from build123d import *

# Parameters (mm, degrees)
ESQUISSE1_W                     = 20
ESQUISSE1_H                     = 40
BOSS_EXTRU_1_DEPTH              = 4
ESQUISSE2_W                     = 19
ESQUISSE2_H                     = 39
ENL_V_MAT_EXTRU_1_DEPTH         = 3.5
ESQUISSE3_W                     = 4.5
ESQUISSE3_H                     = 1.5
BOSS_EXTRU_2_DEPTH              = 4.5
ESQUISSE4_W                     = 4.5
ESQUISSE4_H                     = 1.5
BOSS_EXTRU_3_DEPTH              = 4.5
ESQUISSE5_W                     = 4.5
ESQUISSE5_H                     = 1.5
BOSS_EXTRU_4_DEPTH              = 4.5
ESQUISSE6_W                     = 4.5
ESQUISSE6_H                     = 1.5
BOSS_EXTRU_5_DEPTH              = 4.5
ESQUISSE7_W                     = 4.5
ESQUISSE7_H                     = 1.5
ENL_V_MAT_EXTRU_2_DEPTH         = 4.5
ESQUISSE8_W                     = 4.5
ESQUISSE8_H                     = 1.5
ENL_V_MAT_EXTRU_3_DEPTH         = 4.5
ESQUISSE9_W                     = 4.5
ESQUISSE9_H                     = 1.5
ENL_V_MAT_EXTRU_4_DEPTH         = 4.5
ESQUISSE10_W                    = 4.5
ESQUISSE10_H                    = 1.5
ENL_V_MAT_EXTRU_5_DEPTH         = 4.5
ESQUISSE11_W                    = 6
ESQUISSE11_H                    = 2.5
ENL_V_MAT_EXTRU_6_DEPTH         = 0.25
ESQUISSE12_W                    = 1.25
ESQUISSE12_H                    = 2
ESQUISSE13_W                    = 1.25
ESQUISSE13_H                    = 2
ESQUISSE14_W                    = 1.25
ESQUISSE14_H                    = 2
ESQUISSE15_W                    = 1.25
ESQUISSE15_H                    = 2
DIAM_TRE_DU_PER_AGE_1_5_1_5_1_D = 1.5
CHANFREIN1_SIZE                 = 0.707106781
CHANFREIN2_SIZE                 = 1
CONG_1_R                        = 1.5
CONG_2_R                        = 2
CONG_3_R                        = 2.5
CONG_4_R                        = 3


with BuildPart() as part:
    # Esquisse1 → Boss.-Extru.1 (new body)
    with BuildSketch(Plane(origin=(0, 0, 0), x_dir=(1, 0, 0), z_dir=(0, 1, 0))):
        with Locations((22.084435946, -33.026080306)):
            Rectangle(ESQUISSE1_W, ESQUISSE1_H)
    extrude(amount=-BOSS_EXTRU_1_DEPTH)

    # Esquisse2 → Enl_v. mat.-Extru.1 (cut)
    with BuildSketch(Plane(origin=(0, 0, 0), x_dir=(-1, 0, 0), z_dir=(0, 1, 0))):
        with Locations((-22.084435946, 33.026080306)):
            Rectangle(ESQUISSE2_W, ESQUISSE2_H)
    extrude(amount=-ENL_V_MAT_EXTRU_1_DEPTH, mode=Mode.SUBTRACT)

    # Esquisse3 → Boss.-Extru.2 (add)
    with BuildSketch(Plane(origin=(12.584435946, 0, 0), x_dir=(0, 0, -1), z_dir=(1, 0, 0))):
        with Locations((-15.776080306, -2.75)):
            Rectangle(ESQUISSE3_W, ESQUISSE3_H)
    extrude(amount=BOSS_EXTRU_2_DEPTH)

    # Esquisse4 → Boss.-Extru.3 (add)
    with BuildSketch(Plane.XY.offset(13.526080306)):
        with Locations((29.334435946, -2.75)):
            Rectangle(ESQUISSE4_W, ESQUISSE4_H)
    extrude(amount=BOSS_EXTRU_3_DEPTH)

    # Esquisse5 → Boss.-Extru.4 (add)
    with BuildSketch(Plane(origin=(12.584435946, 0, 0), x_dir=(0, 0, -1), z_dir=(1, 0, 0))):
        with Locations((-50.276080306, -2.75)):
            Rectangle(ESQUISSE5_W, ESQUISSE5_H)
    extrude(amount=BOSS_EXTRU_4_DEPTH)

    # Esquisse6 → Boss.-Extru.5 (add)
    with BuildSketch(Plane(origin=(0, 0, 52.526080306), x_dir=(-1, 0, 0), z_dir=(0, 0, -1))):
        with Locations((-29.334435946, -2.75)):
            Rectangle(ESQUISSE6_W, ESQUISSE6_H)
    extrude(amount=BOSS_EXTRU_5_DEPTH)

    # Esquisse7 → Enl_v. mat.-Extru.2 (cut)
    with BuildSketch(Plane.ZY.offset(-12.084435946)):
        with Locations((15.276080306, -3.25)):
            Rectangle(ESQUISSE7_W, ESQUISSE7_H)
    extrude(amount=-ENL_V_MAT_EXTRU_2_DEPTH, mode=Mode.SUBTRACT)

    # Esquisse8 → Enl_v. mat.-Extru.3 (cut)
    with BuildSketch(Plane(origin=(0, 0, 13.026080306), x_dir=(-1, 0, 0), z_dir=(0, 0, -1))):
        with Locations((-29.834435946, -3.25)):
            Rectangle(ESQUISSE8_W, ESQUISSE8_H)
    extrude(amount=-ENL_V_MAT_EXTRU_3_DEPTH, mode=Mode.SUBTRACT)

    # Esquisse9 → Enl_v. mat.-Extru.4 (cut)
    with BuildSketch(Plane.ZY.offset(-12.084435946)):
        with Locations((50.776080306, -3.25)):
            Rectangle(ESQUISSE9_W, ESQUISSE9_H)
    extrude(amount=-ENL_V_MAT_EXTRU_4_DEPTH, mode=Mode.SUBTRACT)

    # Esquisse10 → Enl_v. mat.-Extru.5 (cut)
    with BuildSketch(Plane(origin=(32.084435946, 0, 0), x_dir=(0, 0, -1), z_dir=(1, 0, 0))):
        with Locations((-50.776080306, -3.25)):
            Rectangle(ESQUISSE10_W, ESQUISSE10_H)
    extrude(amount=-ENL_V_MAT_EXTRU_5_DEPTH, mode=Mode.SUBTRACT)

    # Esquisse11 → Enl_v. mat.-Extru.6 (cut)
    with BuildSketch(Plane.XY.offset(53.026080306)):
        with Locations((22.084435946, -1.25)):
            Rectangle(ESQUISSE11_W, ESQUISSE11_H)
    extrude(amount=-ENL_V_MAT_EXTRU_6_DEPTH, mode=Mode.SUBTRACT)

    # Esquisse12 → R_volution1 (revolve)
    with BuildSketch(Plane.XY.offset(15.026080306), mode=Mode.PRIVATE) as r_volution1_sk:
        with Locations((30.709435946, -1)):
            Rectangle(ESQUISSE12_W, ESQUISSE12_H)
    revolve(r_volution1_sk.sketch.rotate(Axis((30.084435946, 0, 15.026080306), (0, -1, 0)), 270), axis=Axis((30.084435946, 0, 15.026080306), (0, -1, 0)))

    # Esquisse13 → R_volution2 (revolve)
    with BuildSketch(Plane.XY.offset(15.026080306), mode=Mode.PRIVATE) as r_volution2_sk:
        with Locations((14.709435946, -1)):
            Rectangle(ESQUISSE13_W, ESQUISSE13_H)
    revolve(r_volution2_sk.sketch.rotate(Axis((14.084435946, 0, 15.026080306), (0, -1, 0)), 270), axis=Axis((14.084435946, 0, 15.026080306), (0, -1, 0)))

    # Esquisse14 → R_volution3 (revolve)
    with BuildSketch(Plane.XY.offset(51.026080306), mode=Mode.PRIVATE) as r_volution3_sk:
        with Locations((14.709435946, -1)):
            Rectangle(ESQUISSE14_W, ESQUISSE14_H)
    revolve(r_volution3_sk.sketch.rotate(Axis((14.084435946, 0, 51.026080306), (0, -1, 0)), 270), axis=Axis((14.084435946, 0, 51.026080306), (0, -1, 0)))

    # Esquisse15 → R_volution4 (revolve)
    with BuildSketch(Plane.XY.offset(51.026080306), mode=Mode.PRIVATE) as r_volution4_sk:
        with Locations((30.709435946, -1)):
            Rectangle(ESQUISSE15_W, ESQUISSE15_H)
    revolve(r_volution4_sk.sketch.rotate(Axis((30.084435946, 0, 51.026080306), (0, -1, 0)), 270), axis=Axis((30.084435946, 0, 51.026080306), (0, -1, 0)))

    # Diam_tre du per_age _1.5 _1.5_1 (through all)
    with Locations(Plane(origin=(0, -2.5, 0), x_dir=(-1, 0, 0), z_dir=(0, -1, 0))):
        with Locations((-30.084435946, -51.026080306), (-14.084435946, -51.026080306), (-14.084435946, -15.026080306), (-30.084435946, -15.026080306)):
            Hole(DIAM_TRE_DU_PER_AGE_1_5_1_5_1_D / 2)

    # Chanfrein1
    chanfrein1_edges = [part.edges().sort_by_distance(p)[0] for p in [
        (12.584435946, -3.5, 33.026080306),
        (22.084435946, -3.5, 13.526080306),
        (22.084435946, -3.5, 52.526080306),
        (31.584435946, -3.5, 33.026080306),
    ]]
    chamfer(chanfrein1_edges, length=CHANFREIN1_SIZE)

    # Chanfrein2
    chanfrein2_edges = [part.edges().sort_by_distance(p)[0] for p in [
        (22.084435946, -4, 53.026080306),
        (32.084435946, -4, 33.026080306),
        (12.084435946, -4, 33.026080306),
        (22.084435946, -4, 13.026080306),
    ]]
    chamfer(chanfrein2_edges, length=CHANFREIN2_SIZE)

    # Cong_1
    cong_1_edges = [part.edges().sort_by_distance(p)[0] for p in [
        (12.584435946, -1, 13.526080306),
        (31.584435946, -1, 13.526080306),
        (12.584435946, -1, 52.526080306),
        (31.584435946, -1, 52.526080306),
    ]]
    fillet(cong_1_edges, radius=CONG_1_R)

    # Cong_2
    cong_2_edges = [part.edges().sort_by_distance(p)[0] for p in [
        (12.084435946, -1.25, 53.026080306),
        (32.084435946, -1.25, 53.026080306),
        (12.084435946, -1.25, 13.026080306),
        (32.084435946, -1.25, 13.026080306),
    ]]
    fillet(cong_2_edges, radius=CONG_2_R)

    # Cong_3
    cong_3_edges = [part.edges().sort_by_distance(p)[0] for p in [
        (27.584435946, -3.25, 17.526080306),
        (16.584435946, -3.25, 48.526080306),
        (27.584435946, -3.25, 48.526080306),
        (16.584435946, -3.25, 17.526080306),
    ]]
    fillet(cong_3_edges, radius=CONG_3_R)

    # Cong_4
    cong_4_edges = [part.edges().sort_by_distance(p)[0] for p in [
        (17.084435946, -2.75, 18.026080306),
        (27.084435946, -2.75, 18.026080306),
        (17.084435946, -2.75, 48.026080306),
        (27.084435946, -2.75, 48.026080306),
    ]]
    fillet(cong_4_edges, radius=CONG_4_R)


solid = part.part
Verification items for the finished model (mm, model axes). A direction names the side the tool comes from. Give positions to 0.01 mm unless a question says otherwise; leave off trailing zeros. Loops run counter-clockwise (first coordinate to the right, second up) from the corner with the lowest first, then second, coordinate; pieces in that order, holes last. Notation, with made-up numbers: (78.5, 55.25) - (83.5, 55.25) arc R19 cw to (83.5, 87.25) - close; hole circle Ø7 at (-16, 5). An arc over 180 degrees is marked (long way). Write item = value, one per line. Start each with the question number.
Q1. Cross-section at B-B, the plane z = 30. Enter the section's corners in (x, y), and give its area (3 significant figures).
Q2. Mould release check, pull along Z, two halves, no side actions. Record for faces 1 (the face through (22, -1, 13.026)), 2 (the face through (22.007, -3.507, 52.519)), 3 (the face through (17.084, -3, 14)), 4 (the face through (13.012, -1.014, 52.075)): released by +Z, released by -Z, zero draft, split by the parting line, or undercut.
Q3. Cross-section at A-A, the plane y = -0.45. State how many separate pieces and enclosed holes the cut face has, and give its area (3 significant figures).
Q4. Tool access check on faces 5 (the face through (28.297, -3.24, 16.774)), 6 (the face through (15.833, -3.24, 16.813)), 7 (the face through (28.864, -0.986, 15.297)), 8 (the face through (29, -2.5, 51)). Record the directions out of +Z, -Z, +X, -X, +Y, -Y that give a thin tool (end or side, any length) a straight path to the whole face; none if there is none.
Q5. Cross-section at C-C, the plane x = 19.5. Enter the section's corners in (y, z), and give its area (3 significant figures).
Q6. Thickness scan on line 1 (Z direction, x = 21, y = -0.5); line 2 (X direction, y = -0.4, z = 26); line 3 (X direction, y = -0.4, z = 51.5). Record the ranges inside material, lowest first.
Q7. Depth check by flat-ended pin: P1, Ø2, axis at x = 22, z = 43.5, coming from the +Y side; P2, Ø0.8, axis at x = 30.5, y = -3, coming from the +Z side; P3, Ø1.3, axis at x = 15, z = 51.5, coming from the -Y side. Enter the tip coordinate at first touch or a pass-through.
Answer key:
q1.outline = (12.08, -3) - (13.08, -4) - (31.08, -4) - (32.08, -3) - (32.08, 0) - (31.58, 0) - (31.58, -2.79) - (30.88, -3.5) - (13.29, -3.5) - (12.58, -2.79) - (12.58, 0) - (12.08, 0) - close
q1.area = 13.0 mm^2
q2.face_1 = released by -Z
q2.face_2 = released by +Z
q2.face_3 = undercut
q2.face_4 = undercut
q3.separate_pieces = 5
q3.enclosed_holes = 5
q3.area = 68.6 mm^2
q4.face_5 = -Z, +X, -Y
q4.face_6 = -Z, -X, -Y
q4.face_7 = +Y
q4.face_8 = +Z, +X, -Y
q5.outline = (-4, 14.03) - (-3, 13.03) - (0, 13.03) - (0, 13.53) - (-2.79, 13.53) - (-3.5, 14.23) - (-3.5, 51.82) - (-2.79, 52.53) - (0, 52.53) - (0, 52.78) - (-2.5, 52.78) - (-2.5, 53.03) - (-3, 53.03) - (-4, 52.03) - close
q5.area = 22.4 mm^2
q6.line_1 = 13.03 to 13.53, 52.53 to 52.78
q6.line_2 = 12.08 to 12.58, 31.58 to 32.08
q6.line_3 = 12.14 to 12.66, 12.93 to 13.5, 14.67 to 15.24, 28.93 to 29.5, 30.67 to 31.24, 31.51 to 32.03
q7.P1 = -3.5
q7.P2 = 48.53
q7.P3 = -2.5
